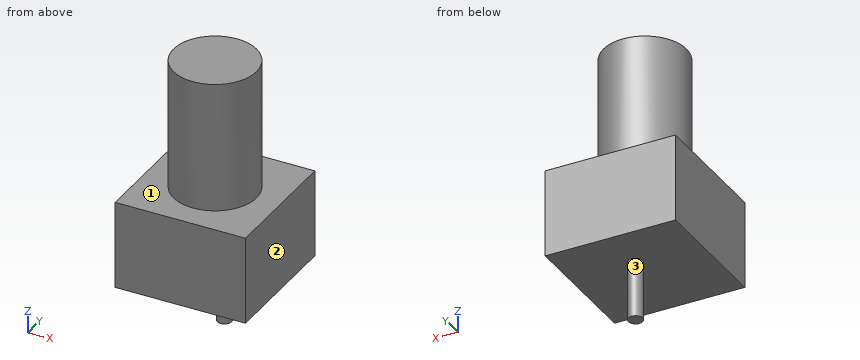
```python
from build123d import *

# Parameters (mm, degrees)
SKETCH1_W           = 55
SKETCH1_H           = 55
BOSS_EXTRUDE1_DEPTH = 37
SKETCH2_R           = 17.5
BOSS_EXTRUDE2_DEPTH = 55
SKETCH3_R           = 3
BOSS_EXTRUDE3_DEPTH = 25


with BuildPart() as part:
    # Sketch1 → Boss-Extrude1 (new body)
    with BuildSketch(Plane.XY):
        Rectangle(SKETCH1_W, SKETCH1_H)
    extrude(amount=BOSS_EXTRUDE1_DEPTH)

    # Sketch2 → Boss-Extrude2 (add)
    with BuildSketch(Plane.XY.offset(37)):
        Circle(SKETCH2_R)
    extrude(amount=BOSS_EXTRUDE2_DEPTH)

    # Sketch3 → Boss-Extrude3 (add)
    with BuildSketch(Plane(origin=(0, 0, 0), x_dir=(-1, 0, 0), z_dir=(0, 0, -1))):
        with Locations(Location((0, 7.5, 0), (0, 0, 180))):
            Circle(SKETCH3_R)
    extrude(amount=BOSS_EXTRUDE3_DEPTH)


solid = part.part
```
CAD build for the part. Positions are in the model's coordinates, mm. Face numbers are marked on the shaded views. A direction names the side the tool comes from. Give positions to 0.01 mm unless a question says otherwise; leave off trailing zeros. Order: outer loops, then holes, each group sorted by start corner. A loop starts at its lowest first (then second) coordinate and runs counter-clockwise, first axis right, second up.
(1) Saw through at C-C, the plane z = 62.5. Give the cut face in (x, y).
(2) Tool access for the marked faces 1, 2 and 3: list every direction of +Z, -Z, +X, -X, +Y, -Y with a clear straight run to the whole face (end or side of a thin tool).
(3) Saw through at D-D, the plane y = -10. Give the cut face in (x, z).
(4) Saw through at A-A, the plane y = 0. Give the cut face in (x, z).
(5) Flat gauge pins, fed straight in: pin 1 (2 mm diameter, centred on y = -10, z = 58, fed in from -X); pin 2 (12 mm diameter, centred on x = -12, y = 21.5, fed in from -Z); pin 3 (12 mm diameter, centred on x = -10.5, z = -13, fed in from -Y). Where does each tip first touch, or does it go through?
(6) Saw through at B-B, the plane x = 0. Give the cut face in (y, z).
(7) Drill centre lines: L1, parallel to Z at x = 15, y = 10.5; L2, parallel to Z at x = 2, y = -12.5; L3, parallel to X at y = 4, z = 37.5. Where is each one in solid material? Low to high.
Results found:
1. outline: circle Ø35 at (0, 0)
2. face 1: +Z
2. face 2: +Z, -Z, +X, +Y, -Y
2. face 3: -Z
3. outline: (-27.5, 0) - (27.5, 0) - (27.5, 37) - (14.36, 37) - (14.36, 92) - (-14.36, 92) - (-14.36, 37) - (-27.5, 37) - close
4. outline: (-27.5, 0) - (27.5, 0) - (27.5, 37) - (17.5, 37) - (17.5, 92) - (-17.5, 92) - (-17.5, 37) - (-27.5, 37) - close
5. pin 1: stops at x = -15.01
5. pin 2: stops at z = 0
5. pin 3: passes through
6. outline: (-27.5, 0) - (4.5, 0) - (4.5, -25) - (10.5, -25) - (10.5, 0) - (27.5, 0) - (27.5, 37) - (17.5, 37) - (17.5, 92) - (-17.5, 92) - (-17.5, 37) - (-27.5, 37) - close
7. L1: z = 0 to 37
7. L2: z = 0 to 92
7. L3: x = -17.04 to 17.04
